Build history of the part. All positions in model axes, mm. Round coordinates to 2 decimals unless told otherwise and drop trailing zeros. Order: outer loops, then holes, each group sorted by start corner. A loop starts at its lowest first (then second) coordinate and runs counter-clockwise, first axis right, second up. Notation, with made-up numbers: (88, -23.75) -> (112, -23.75) arc R30 cw to (112, 13.25) -> close; hole circle Ø6 at (33, -32). An arc over 180 degrees is marked (long way). Write item = value, one per line.
from build123d import *

# Parameters (mm, degrees)
SKETCH1_R           = 3
BOSS_EXTRUDE1_DEPTH = 7
FILLET2_R           = 0.2
FILLET3_R           = 0.2


with BuildPart() as part:
    # Sketch1 → Boss-Extrude1 (new body)
    with BuildSketch(Plane.XY):
        with Locations(Location((0, 0, 0), (0, 0, 180))):
            Circle(SKETCH1_R)
    extrude(amount=BOSS_EXTRUDE1_DEPTH)

    # Fillet2
    fillet2_edges = [part.edges().sort_by_distance(p)[0] for p in [
        (3, 0, 7),
    ]]
    fillet(fillet2_edges, radius=FILLET2_R)

    # Fillet3
    fillet3_edges = [part.edges().sort_by_distance(p)[0] for p in [
        (3, 0, 0),
    ]]
    fillet(fillet3_edges, radius=FILLET3_R)

    # Sketch4 → Revolve1 (revolve)
    with BuildSketch(Plane(origin=(0, 0, 0), x_dir=(1, 0, 0), z_dir=(0, 1, 0))):
        with BuildLine():
            Line((0, 0), (2.8, 0))
            Line((2.8, 0), (0.348733134, 1.30569363))
            ThreePointArc((0.348733134, 1.30569363), (0.479948636, 1.872008824), (0, 2.200002288))
            Line((0, 2.200002288), (0, 0))
        make_face()
    revolve(axis=Axis((0, 0, -5.421968799), (0, 0, 1)))


solid = part.part
Q1. Flat gauge pins, fed straight in: pin 1 (1.5 mm diameter, centred on x = 2.5, z = 2.5, fed in from -Y); pin 2 (2 mm diameter, centred on x = -2.5, y = -1.5, fed in from -Z). Where does each tip first touch, or does it go through?
Check values:
pin_1 = -2.44
pin_2 = -0.47
Q2. Cut at C-C, the plane z = 2.75. List the corners of the cut face in (x, y).
Check values:
outline = circle Ø6 at (0, 0)
Q3. Probe probe 1 along Z at (x, y) = (-1.25, -1.75); probe 2 along X at (y, z) = (2.75, 4.5); probe 3 along Y at (x, z) = (-1.75, 4). List the from-to ranges inside material, lowest first.
Check values:
probe_1 = -0.35 to 7
probe_2 = -1.2 to 1.2
probe_3 = -2.44 to 2.44
Q4. Cut at A-A, the plane y = 0. List the corners of the cut face in (x, z).
Check values:
outline = (-3, 0.2) arc R0.2 ccw to (-2.8, 0) -> (-0.35, -1.31) arc R0.52 ccw (long way) to (0.35, -1.31) -> (2.8, 0) arc R0.2 ccw to (3, 0.2) -> (3, 6.8) arc R0.2 ccw to (2.8, 7) -> (-2.8, 7) arc R0.2 ccw to (-3, 6.8) -> close
Q5. Cut at D-D, the plane z = -0.5. List the corners of the cut face in (x, y), and give its area (3 significant figures).
Check values:
outline = circle Ø3.72 at (0, 0)
area = 10.9 mm²
